from build123d import *

# Parameters (mm, degrees)
BOSS_EXTRUDE1_DEPTH = 40
SKETCH4_W           = 6
SKETCH4_H           = 40
CUT_EXTRUDE1_DEPTH  = 4.7625
SKETCH5_R           = 4
SKETCH5_R_2         = 2
CUT_EXTRUDE2_DEPTH  = 4.7625


with BuildPart() as part:
    # Sketch3 → Boss-Extrude1 (new body)
    with BuildSketch(Plane.XY):
        Polygon((26.19375, -9.525), (26.19375, -14.2875), (-2.38125, -14.2875), (-2.38125, 9.525), (-26.19375, 9.525), (-26.19375, 14.2875), (2.38125, 14.2875), (2.38125, -9.525), align=None)
    extrude(amount=BOSS_EXTRUDE1_DEPTH)

    # Sketch4 → Cut-Extrude1 (cut)
    with BuildSketch(Plane(origin=(0, 14.2875, 0), x_dir=(1, 0, 0), z_dir=(0, 1, 0))):
        with Locations((-23.19375, -20)):
            Rectangle(SKETCH4_W, SKETCH4_H)
    extrude(amount=-CUT_EXTRUDE1_DEPTH, mode=Mode.SUBTRACT)

    # Sketch5 → Cut-Extrude2 (cut)
    with BuildSketch(Plane.XZ.offset(14.2875)):
        with Locations(Location((11.19375, 7.5, 0), (0, 0, 270))):
            Circle(SKETCH5_R)
        with Locations(Location((11.19375, 22.5, 0), (0, 0, 270))):
            Circle(SKETCH5_R)
        with Locations(Location((22.0033493, 35.1973816, 0), (0, 0, 270))):
            Circle(SKETCH5_R_2)
    extrude(amount=-CUT_EXTRUDE2_DEPTH, mode=Mode.SUBTRACT)


solid = part.part
Geometry check sheet. Reference: the model listing, model coordinates, mm. A direction names the side the tool comes from. Round coordinates to 2 decimals unless told otherwise and drop trailing zeros. Loops run counter-clockwise (first coordinate to the right, second up) from the corner with the lowest first, then second, coordinate; pieces in that order, holes last.
Item 1: Thickness scan on line 1 (X direction, y = -12.4, z = 7.5); line 2 (X direction, y = 0, z = 27.5); line 3 (Y direction, x = 15, z = 15.5) (1 decimal). Record the ranges inside material, lowest first.
Item 2: Access from +Z, -Z, +X, -X, +Y, -Y to the whole of each face (thin tool, end or side, straight path). Record for faces 1 (the flat face through (2.381, 3, 20)), 2 (the flat face through (-11, 9.525, 20)), 3 (the flat face through (15, -14.288, 20)).
Item 3: Mould release check, pull along X, two halves, no side actions. Record for faces 4 (the flat face through (-2.381, -3, 20)), 5 (the cylindrical face through (8.76, -11.94, 25.674)), 6 (the flat face through (1, -1, 40)): pulls with the +X half, pulls with the -X half, needs draft (parallel to the pull), parting line crosses it, or undercut.
Item 4: Cross-section at A-A on z = 7.5. Record the boundary of the cut face in (x, y) (1 decimal), then the cut area to 3 significant figures.
Item 5: Cross-section at B-B on z = 17.5. Record the boundary of the cut face in (x, y) (1 decimal), then the cut area to 3 significant figures.
Item 6: Cross-section at C-C on x = 19. Record the boundary of the cut face in (y, z) (1 decimal), then the cut area to 4 significant figures.
Item 7: Gauge pin test, flat ends, axial feed: pin 1 (7 mm diameter, centred on x = 17.5, z = 23.5, fed in from +Y) (3 decimals); pin 2 (6 mm diameter, centred on y = 7.5, z = 19, fed in from +X); pin 3 (12 mm diameter, centred on y = 2, z = 14, fed in from -X); pin 4 (2.5 mm diameter, centred on x = 22, z = 35.2, fed in from -Y). Record the tip position at first contact, or that the pin passes through.
Item 8: Cross-section at D-D on y = -4. Record the boundary of the cut face in (x, z), then the cut area to 4 significant figures.
Answer sheet:
1. line 1: x = -2.38 to 7.19, 15.19 to 26.19
1. line 2: x = -2.38 to 2.38
1. line 3: y = -14.3 to -9.5
2. face 1: +Z, -Z, +X, +Y
2. face 2: +Z, -Z, -X, -Y
2. face 3: +Z, -Z, +X, -X, -Y
3. face 4: pulls with the -X half
3. face 5: undercut
3. face 6: needs draft
4. outline: (-20.2, 9.5) - (-2.4, 9.5) - (-2.4, -14.3) - (7.2, -14.3) - (7.2, -9.5) - (2.4, -9.5) - (2.4, 14.3) - (-20.2, 14.3) - close; (15.2, -14.3) - (26.2, -14.3) - (26.2, -9.5) - (15.2, -9.5) - close
4. area: 296 mm2
5. outline: (-20.2, 9.5) - (-2.4, 9.5) - (-2.4, -14.3) - (26.2, -14.3) - (26.2, -9.5) - (2.4, -9.5) - (2.4, 14.3) - (-20.2, 14.3) - close
5. area: 334 mm2
6. outline: (-14.3, 0) - (-9.5, 0) - (-9.5, 40) - (-14.3, 40) - close
6. area: 190.5 mm2
7. pin 1: stops at y = -9.525
7. pin 2: stops at x = 2.38
7. pin 3: stops at x = -2.38
7. pin 4: passes through
8. outline: (-2.38, 0) - (2.38, 0) - (2.38, 40) - (-2.38, 40) - close
8. area: 190.5 mm2
